```python
from build123d import *

# Parameters (mm, degrees)
SKETCH1_R           = 38.1
BOSS_EXTRUDE1_DEPTH = 25.4
SKETCH2_W           = 50.8
SKETCH2_H           = 20.32
BOSS_EXTRUDE2_DEPTH = 50.8
CUT_EXTRUDE1_REACH  = 87.194
SKETCH3_R           = 3.81


with BuildPart() as part:
    # Sketch1 → Boss-Extrude1 (new body)
    with BuildSketch(Plane(origin=(0, 0, 0), x_dir=(1, 0, 0), z_dir=(0, 1, 0))):
        with Locations(Location((0, 0, 0), (0, 0, 270))):
            Circle(SKETCH1_R)
    extrude(amount=BOSS_EXTRUDE1_DEPTH)

    # Sketch2 → Boss-Extrude2 (add)
    with BuildSketch(Plane.XY):
        with Locations((0, 12.7)):
            Rectangle(SKETCH2_W, SKETCH2_H)
    extrude(amount=BOSS_EXTRUDE2_DEPTH)

    # Sketch3 → Cut-Extrude1 (cut, up to next)
    with BuildSketch(Plane.ZY.offset(25.4), mode=Mode.PRIVATE) as cut_extrude1_sk1:
        with Locations(Location((39.599031657, 12.7, 0), (0, 0, 270))):
            Circle(SKETCH3_R)
    cut_extrude1_tool1 = extrude(cut_extrude1_sk1.sketch, amount=-CUT_EXTRUDE1_REACH, mode=Mode.PRIVATE) & part.part
    add(cut_extrude1_tool1.solids().sort_by_distance((-25.4, 12.7, 39.599032))[0], mode=Mode.SUBTRACT)


solid = part.part
```
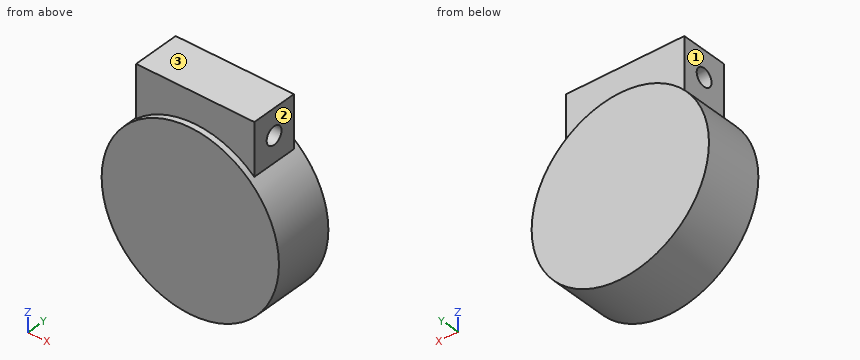
Design review of the part built by this model. Coordinates are the model's own, in mm. Face numbers are marked on the shaded views. A direction names the side the tool comes from. Round coordinates to 2 decimals unless told otherwise and drop trailing zeros. Write each loop counter-clockwise with the first axis right and the second up, starting at its lowest first coordinate (ties: lowest second). Pieces come first, ordered by that corner, then holes. Notation, with made-up numbers: (36.5, 22) -> (59.5, 22) arc R9 cw to (59.5, 31) -> close; hole circle Ø8 at (54, -14.75). An arc over 180 degrees is marked (long way). Answer in a Markdown table with one row per item.
Q1. Clearance check with flat-ended pins moving along their axes: pin 1 Ø1.5 at (y, z) = (18, 31) entering from +X; pin 2 Ø3 at (y, z) = (19.5, -11) entering from -X; pin 3 Ø4 at (x, y) = (4.5, 5) entering from -Z. State where each tip first meets the part, or that it passes through.
The answers:
| item | result |
|---|---|
| pin 1 | x = 25.4 |
| pin 2 | x = -36.9 |
| pin 3 | z = -38.02 |
Q2. Take a section at C-C, the plane y = 5. State the section outline as (x, z) points, then the cut area to 3 significant figures.
The answers:
| item | result |
|---|---|
| outline | (-25.4, 28.4) arc R38.1 ccw (long way) to (25.4, 28.4) -> (25.4, 50.8) -> (-25.4, 50.8) -> close |
| area | 5,360 mm² |
Q3. Take a section at A-A, the plane y = 12.7. State the section outline as (x, z) points, then the cut area to 3 significant figures.
The answers:
| item | result |
|---|---|
| outline | (-25.4, 28.4) arc R38.1 ccw (long way) to (25.4, 28.4) -> (25.4, 35.79) -> (-25.4, 35.79) -> close; (-25.4, 43.41) -> (25.4, 43.41) -> (25.4, 50.8) -> (-25.4, 50.8) -> close |
| area | 4,970 mm² |
Q4. To check wall thickness, follow L1, parallel to Y at x = -8, z = 39.5; L2, parallel to Y at x = -18, z = 36.5; L3, parallel to Z at x = -15.5, y = 12. State the ranges of each line that lie inside material, in increasing order. Write a range as [from, to].
The answers:
| item | result |
|---|---|
| L1 | [2.54, 8.89], [16.51, 22.86] |
| L2 | [2.54, 10.48], [14.92, 22.86] |
| L3 | [-34.8, 35.85], [43.34, 50.8] |
Q5. Take a section at D-D, the plane x = 19. State the section outline as (y, z) points.
The answers:
| item | result |
|---|---|
| outline | (0, -33.02) -> (25.4, -33.02) -> (25.4, 33.02) -> (22.86, 33.02) -> (22.86, 50.8) -> (2.54, 50.8) -> (2.54, 33.02) -> (0, 33.02) -> close; hole circle Ø7.62 at (12.7, 39.6) |
Q6. For the marked faces 1, 2 and 3, list the 3-axis set-ups (+Z, -Z, +X, -X, +Y, -Y) from which the entire face can be reached by the end or side of a thin tool; tool diameter is ignored.
The answers:
| item | result |
|---|---|
| face 1 | +Z, -X, +Y, -Y |
| face 2 | +Z, +X, +Y, -Y |
| face 3 | +Z, +X, -X, +Y, -Y |
Q7. Take a section at B-B, the plane x = 0. State the section outline as (y, z) points.
The answers:
| item | result |
|---|---|
| outline | (0, -38.1) -> (25.4, -38.1) -> (25.4, 38.1) -> (22.86, 38.1) -> (22.86, 50.8) -> (2.54, 50.8) -> (2.54, 38.1) -> (0, 38.1) -> close; hole circle Ø7.62 at (12.7, 39.6) |
